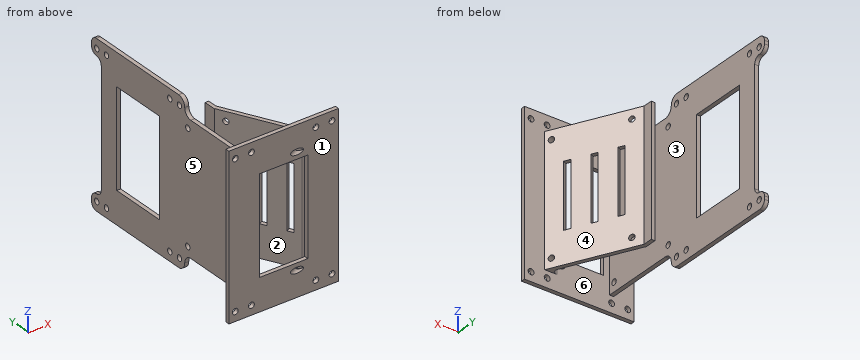
```python
from build123d import *

# Parameters (mm, degrees)
SKETCH_1_W           = 68
SKETCH_1_H           = 100
SKETCH_1_R           = 1.8
EXTRUDE_1_DEPTH      = 2.5
SKETCH_3_W           = 2.5
SKETCH_3_H           = 80
EXTRUDE_2_DEPTH      = 55
SKETCH_4_W           = 30
SKETCH_4_H           = 60
CUT_EXTRUDE_1_DEPTH  = 55
EXTRUDE_3_DEPTH      = 40
EXTRUDE_3_DEPTH_BACK = 40
SKETCH_5_W           = 80
SKETCH_5_H           = 55
EXTRUDE_5_DEPTH      = 2.5
SKETCH_6_R           = 1.8
CUT_EXTRUDE_2_DEPTH  = 2.5
SKETCH_7_R           = 1.8
CUT_EXTRUDE_3_DEPTH  = 2.5
EXTRUDE_START        = 55
SKETCH_8_W           = 2.236067978
SKETCH_8_H           = 80
EXTRUDE_6_DEPTH      = 7.5
SKETCH_10_R          = 1.8
SKETCH_10_W          = 80
SKETCH_10_H          = 3
SKETCH_10_W_2        = 10
SKETCH_10_H_2        = 1.3
SKETCH_10_W_3        = 100
EXTRUDE_7_DEPTH      = 2.5
FILLET_1_R           = 5
FILLET_4_R           = 3
SKETCH_11_R          = 1.8
CUT_EXTRUDE_4_DEPTH  = 30
SKETCH_13_W          = 40
SKETCH_13_H          = 4
CUT_EXTRUDE_5_DEPTH  = 2.5
SKETCH_14_R          = 1.8
CUT_EXTRUDE_6_DEPTH  = 2.5
SKETCH_15_R          = 1.8
EXTRUDE_10_DEPTH     = 2.5
FILLET_6_R           = 4
SKETCH_16_W          = 60
SKETCH_16_H          = 35.254237288
CUT_EXTRUDE_8_DEPTH  = 10


# Some blends are built 0.0001 mm under size
with BuildPart() as part:
    # 草图1 → 凸台-拉伸1 (new body)
    with BuildSketch(Plane(origin=(0, 0, 0), x_dir=(1, 0, 0), z_dir=(0, 1, 0))):
        Rectangle(SKETCH_1_W, SKETCH_1_H)
        with Locations(Location((-30, 44.25, 0), (0, 0, 270))):
            Circle(SKETCH_1_R, mode=Mode.SUBTRACT)
        with Locations(Location((30, 44.25, 0), (0, 0, 270))):
            Circle(SKETCH_1_R, mode=Mode.SUBTRACT)
        with Locations(Location((30, -44.25, 0), (0, 0, 270))):
            Circle(SKETCH_1_R, mode=Mode.SUBTRACT)
        with Locations(Location((-30, -44.25, 0), (0, 0, 270))):
            Circle(SKETCH_1_R, mode=Mode.SUBTRACT)
        with Locations(Location((20, -44.25, 0), (0, 0, 270))):
            Circle(SKETCH_1_R, mode=Mode.SUBTRACT)
        with Locations(Location((20, 44.25, 0), (0, 0, 270))):
            Circle(SKETCH_1_R, mode=Mode.SUBTRACT)
        with Locations(Location((-20, -44.25, 0), (0, 0, 270))):
            Circle(SKETCH_1_R, mode=Mode.SUBTRACT)
        with Locations(Location((-20, 44.25, 0), (0, 0, 270))):
            Circle(SKETCH_1_R, mode=Mode.SUBTRACT)
    extrude(amount=EXTRUDE_1_DEPTH)

    # 草图3 → 凸台-拉伸2 (add)
    with BuildSketch(Plane(origin=(0, 2.5, 0), x_dir=(1, 0, 0), z_dir=(0, 1, 0))):
        with Locations((-20, 0)):
            Rectangle(SKETCH_3_W, SKETCH_3_H)
    extrude(amount=EXTRUDE_2_DEPTH)

    # 草图4 → 切除-拉伸1 (cut)
    with BuildSketch(Plane(origin=(0, 2.5, 0), x_dir=(1, 0, 0), z_dir=(0, 1, 0))):
        Rectangle(SKETCH_4_W, SKETCH_4_H)
    extrude(amount=-CUT_EXTRUDE_1_DEPTH, mode=Mode.SUBTRACT)

    # 草图2 → 凸台-拉伸3 (add, two sides: drawn at the far end of the back side and taken through both)
    with BuildSketch(Plane.XY.offset(-EXTRUDE_3_DEPTH_BACK)):
        Polygon((20, 2.5), (21.5, 2.5), (20, 5.5), align=None)
    extrude(amount=EXTRUDE_3_DEPTH + EXTRUDE_3_DEPTH_BACK)

    # 草图5 → 凸台-拉伸5 (add)
    with BuildSketch(Plane(origin=(18.2, 9.1, 0), x_dir=(0, 0, -1), z_dir=(0.8944271909999156, 0.44721359549995837, 0))):
        with Locations((0, 20.120975674)):
            Rectangle(SKETCH_5_W, SKETCH_5_H)
    extrude(amount=-EXTRUDE_5_DEPTH)

    # 草图6 → 切除-拉伸2 (cut)
    with BuildSketch(Plane.ZY.offset(21.25)):
        with Locations((34.25, 50.7)):
            Circle(SKETCH_6_R)
        with Locations((34.25, 6.2)):
            Circle(SKETCH_6_R)
        with Locations((-34.25, 50.7)):
            Circle(SKETCH_6_R)
        with Locations((-34.25, 6.2)):
            Circle(SKETCH_6_R)
    extrude(amount=-CUT_EXTRUDE_2_DEPTH, mode=Mode.SUBTRACT)

    # 草图7 → 切除-拉伸3 (cut)
    with BuildSketch(Plane(origin=(18.2, 9.1, 0), x_dir=(0, 0, -1), z_dir=(0.8944271909999156, 0.44721359549995837, 0))):
        with Locations(Location((34.25, 40.820975674, 0), (0, 0, 90))):
            Circle(SKETCH_7_R)
        with Locations(Location((-34.25, 40.820975674, 0), (0, 0, 90))):
            Circle(SKETCH_7_R)
        with Locations(Location((-34.25, -3.679024326, 0), (0, 0, 90))):
            Circle(SKETCH_7_R)
        with Locations(Location((34.25, -3.679024326, 0), (0, 0, 90))):
            Circle(SKETCH_7_R)
    extrude(amount=-CUT_EXTRUDE_3_DEPTH, mode=Mode.SUBTRACT)

    # 草图8 → 凸台-拉伸6 (add)
    with BuildSketch(Plane(origin=(0, 2.5, 0), x_dir=(1, 0, 0), z_dir=(0, 1, 0)).offset(EXTRUDE_START)):
        with Locations((-4.214781741, 0)):
            Rectangle(SKETCH_8_W, SKETCH_8_H)
    extrude(amount=-EXTRUDE_6_DEPTH)

    # 草图10 → 凸台-拉伸7 (add)
    # profile 1 of 5: a face of its own
    with BuildSketch(Plane.ZY.offset(21.25)):
        Polygon((50, 120.5), (-50, 120.5), (-50, 54.5), (-40, 54.5), (-40, 57.5), (40, 57.5), (40, 54.5), (50, 54.5), align=None)
        with Locations((-44.25, 57.5)):
            Circle(SKETCH_10_R, mode=Mode.SUBTRACT)
        with Locations((44.25, 57.5)):
            Circle(SKETCH_10_R, mode=Mode.SUBTRACT)
        with Locations((-44.25, 117.5)):
            Circle(SKETCH_10_R, mode=Mode.SUBTRACT)
        with Locations((44.25, 117.5)):
            Circle(SKETCH_10_R, mode=Mode.SUBTRACT)
    # profile 2 of 5: a face of its own
    with BuildSketch(Plane.ZY.offset(21.25)):
        with Locations((0, 56)):
            Rectangle(SKETCH_10_W, SKETCH_10_H)
    # profile 3 of 5: a face of its own
    with BuildSketch(Plane.ZY.offset(21.25)):
        with Locations((-45, 53.85)):
            Rectangle(SKETCH_10_W_2, SKETCH_10_H_2)
    # profile 4 of 5: a face of its own
    with BuildSketch(Plane.ZY.offset(21.25)):
        with Locations((45, 53.85)):
            Rectangle(SKETCH_10_W_2, SKETCH_10_H_2)
    # profile 5 of 5: a face of its own
    with BuildSketch(Plane.ZY.offset(21.25)):
        with Locations((0, 121.15)):
            Rectangle(SKETCH_10_W_3, SKETCH_10_H_2)
    extrude(amount=-EXTRUDE_7_DEPTH)

    # 圆角1
    fillet_1_edges = [part.edges().sort_by_distance(p)[0] for p in [
        (-20, 121.8, -50),
        (-20, 121.8, 50),
        (-20, 53.2, 50),
        (-20, 53.2, -50),
        (-20, 53.2, -40),
        (-20, 53.2, 40),
    ]]
    fillet(fillet_1_edges, radius=FILLET_1_R - 0.0001)  # a hair under: the kernel refuses the full size

    # 圆角4
    # the kernel refuses this fillet: 3 mm, written as the material it adds along each edge
    with BuildSketch(Plane(origin=(18.704915028, 2.5, 40), x_dir=(-1, 0, 0), z_dir=(0, 0, -1))) as fillet_4_piece_1_section:
        with BuildLine():
            CenterArc((FILLET_4_R * 1.61803398875, FILLET_4_R), FILLET_4_R, 153.434948823, 116.565051177)
            Line((FILLET_4_R * 0.72360679775, FILLET_4_R * 1.4472135955), (0, 0))
            Line((0, 0), (FILLET_4_R * 1.61803398875, 0))
        make_face()
    fillet_4_piece_1 = extrude(amount=92.135254916, mode=Mode.PRIVATE)
    fillet_4_piece_1 = split(fillet_4_piece_1, bisect_by=Plane(origin=(14.716283271, 2.568197863, 30), z_dir=(0, 0, 1)), keep=Keep.TOP, mode=Mode.PRIVATE)
    fillet_4_piece_1 = fillet_4_piece_1 - Plane(origin=(14.445615458, 3.109533488, 34.25), x_dir=(-0.44721359549995837, 0.8944271909999156, 0), z_dir=(0.8944271909999156, 0.44721359549995837, 0)) * Cylinder(1.8, 204, mode=Mode.PRIVATE)
    add(fillet_4_piece_1)
    with BuildSketch(Plane(origin=(18.704915028, 2.5, 52.135254916), x_dir=(-1, 0, 0), z_dir=(0, 0, -1))) as fillet_4_piece_2_section:
        with BuildLine():
            CenterArc((FILLET_4_R * 1.61803398875, FILLET_4_R), FILLET_4_R, 153.434948823, 116.565051177)
            Line((FILLET_4_R * 0.72360679775, FILLET_4_R * 1.4472135955), (0, 0))
            Line((0, 0), (FILLET_4_R * 1.61803398875, 0))
        make_face()
    fillet_4_piece_2 = extrude(amount=92.135254916, mode=Mode.PRIVATE)
    fillet_4_piece_2 = split(fillet_4_piece_2, bisect_by=Plane(origin=(17.041037704, 3.56720979, 30), z_dir=(0, 0, -1)), keep=Keep.TOP, mode=Mode.PRIVATE)
    fillet_4_piece_2 = split(fillet_4_piece_2, bisect_by=Plane(origin=(15, 3.56720979, 0), z_dir=(1, 0, 0)), keep=Keep.TOP, mode=Mode.PRIVATE)
    fillet_4_piece_2 = fillet_4_piece_2 - Plane(origin=(16.705023776, 4.239237646, -34.25), x_dir=(-0.44721359549995837, 0.8944271909999156, 0), z_dir=(0.8944271909999156, 0.44721359549995837, 0)) * Cylinder(1.8, 204, mode=Mode.PRIVATE)
    add(fillet_4_piece_2)
    with BuildSketch(Plane(origin=(18.704915028, 2.5, 52.135254916), x_dir=(-1, 0, 0), z_dir=(0, 0, -1))) as fillet_4_piece_3_section:
        with BuildLine():
            CenterArc((FILLET_4_R * 1.61803398875, FILLET_4_R), FILLET_4_R, 153.434948823, 116.565051177)
            Line((FILLET_4_R * 0.72360679775, FILLET_4_R * 1.4472135955), (0, 0))
            Line((0, 0), (FILLET_4_R * 1.61803398875, 0))
        make_face()
    fillet_4_piece_3 = extrude(amount=92.135254916, mode=Mode.PRIVATE)
    fillet_4_piece_3 = split(fillet_4_piece_3, bisect_by=Plane(origin=(14.716283305, 2.568197867, -30), z_dir=(0, 0, -1)), keep=Keep.TOP, mode=Mode.PRIVATE)
    fillet_4_piece_3 = fillet_4_piece_3 - Plane(origin=(14.445615487, 3.109533502, -34.25), x_dir=(-0.44721359549995837, 0.8944271909999156, 0), z_dir=(0.8944271909999156, 0.44721359549995837, 0)) * Cylinder(1.8, 204, mode=Mode.PRIVATE)
    add(fillet_4_piece_3)

    # 草图11 → 切除-拉伸4 (cut)
    with BuildSketch(Plane(origin=(18.2, 9.1, 0), x_dir=(0, 0, -1), z_dir=(0.8944271909999156, 0.44721359549995837, 0))):
        with Locations(Location((-34.25, -3.679024326, 0), (0, 0, 90))):
            Circle(SKETCH_11_R)
        with Locations(Location((34.25, -3.679024326, 0), (0, 0, 90))):
            Circle(SKETCH_11_R)
    extrude(amount=-CUT_EXTRUDE_4_DEPTH, mode=Mode.SUBTRACT)

    # 草图13 → 切除-拉伸5 (cut)
    with BuildSketch(Plane(origin=(18.2, 9.1, 0), x_dir=(0, 0, -1), z_dir=(0.8944271909999156, 0.44721359549995837, 0))):
        with Locations((0, 20.120975674)):
            Rectangle(SKETCH_13_W, SKETCH_13_H)
        with Locations((0, 35.120975674)):
            Rectangle(SKETCH_13_W, SKETCH_13_H)
        with Locations((0, 5.120975674)):
            Rectangle(SKETCH_13_W, SKETCH_13_H)
    extrude(amount=-CUT_EXTRUDE_5_DEPTH, mode=Mode.SUBTRACT)

    # 草图14 → 切除-拉伸6 (cut)
    with BuildSketch(Plane.ZY.offset(21.25)):
        with Locations((-44.25, 65.5)):
            Circle(SKETCH_14_R)
        with Locations((44.25, 65.5)):
            Circle(SKETCH_14_R)
    extrude(amount=-CUT_EXTRUDE_6_DEPTH, mode=Mode.SUBTRACT)

    # 草图15 → 凸台-拉伸10 (add)
    # profile 1 of 4: a face of its own
    with BuildSketch(Plane.ZY.offset(21.25)):
        Polygon((-42.960162103, 121.8), (-40, 121.8), (-40, 129.8), (-50, 129.8), (-50, 121.8), (-45, 121.8), align=None)
        with Locations((-44.25, 125.5)):
            Circle(SKETCH_15_R, mode=Mode.SUBTRACT)
    # profile 2 of 4: a face of its own
    with BuildSketch(Plane.ZY.offset(21.25)):
        Polygon((40, 129.8), (40, 121.8), (44.25, 121.8), (45, 121.8), (50, 121.8), (50, 129.8), align=None)
        with Locations((44.25, 125.5)):
            Circle(SKETCH_15_R, mode=Mode.SUBTRACT)
    # profile 3 of 4: a face of its own
    with BuildSketch(Plane.ZY.offset(21.25)):
        Polygon((-50, 114.760162103), (-42.960162103, 121.8), (-45, 121.8), (-50, 121.8), align=None)
    # profile 4 of 4: a face of its own
    with BuildSketch(Plane.ZY.offset(21.25)):
        Polygon((45, 121.8), (44.25, 121.8), (50, 115.456159587), (50, 121.8), align=None)
    extrude(amount=-EXTRUDE_10_DEPTH)

    # 圆角6
    fillet_6_edges = [part.edges().sort_by_distance(p)[0] for p in [
        (-20, 121.8, 40),
        (-20, 129.8, 40),
        (-20, 129.8, 50),
        (-20, 129.8, -50),
        (-20, 129.8, -40),
        (-20, 121.8, -40),
    ]]
    fillet(fillet_6_edges, radius=FILLET_6_R - 0.0001)  # a hair under: the kernel refuses the full size

    # 草图16 → 切除-拉伸8 (cut)
    with BuildSketch(Plane.ZY.offset(21.25)):
        with Locations((0, 91.5)):
            Rectangle(SKETCH_16_W, SKETCH_16_H)
    extrude(amount=-CUT_EXTRUDE_8_DEPTH, mode=Mode.SUBTRACT)


solid = part.part
```
Here's how the part is built. I have some questions about the finished solid (model axes, mm). Face numbers are marked on the shaded views. A direction names the side the tool comes from. Give positions to 0.01 mm unless a question says otherwise; leave off trailing zeros. Order: outer loops, then holes, each group sorted by start corner. A loop starts at its lowest first (then second) coordinate and runs counter-clockwise, first axis right, second up. Notation, with made-up numbers: (-38, 42.5) -> (-32, 42.5) arc R27 cw to (-32, 67.5) -> close; hole circle Ø8 at (-10.5, -29.75). An arc over 180 degrees is marked (long way). Use CSV: the item, a comma, the result in double quotes. Start each with the question number.
Item 1: Thinking about a two-plate mould opening in X: for the marked faces 4, 5 and 6, which applies, pulls with the +X half, pulls with the -X half, needs draft (parallel to the pull), parting line crosses it, or undercut?
Item 2: Suppose I cut it at B-B (y = 84.5). List the corners of the cut face in (x, z) for me.
Item 3: Suppose I cut it at D-D (y = 65.5). List the corners of the cut face in (x, z) for me, and give its area (3 significant figures).
Item 4: I'm going to push flat-ended pins straight in: P1, Ø2, axis at y = 112, z = -25, coming from the -X side; P2, Ø2.5, axis at x = -3.5, z = 7.5, coming from the +Y side; P3, Ø4.5, axis at x = 14, y = 12, coming from the +Z side. Where does each tip first touch, or does it pass through?
Item 5: If I drill on probe 1 along X at (y, z) = (1.1, -44.25); probe 2 along Y at (x, z) = (-19.55, -34.25); probe 3 along Z at (x, y) = (-20.6, 117.5), over which ranges is the centre line in solid material (lowest first)? Write a range as [from, to].
Item 6: Suppose I cut it at A-A (x = -11). List the corners of the cut face in (y, z) for me.
Item 7: On a 3-axis mill with a long thin cutter (end or side, diameter ignored), from which of +Z, -Z, +X, -X, +Y, -Y can I reach the whole of each face in a straight line? I mean the marked faces 1, 2 and 3. Say none if no direction works.
Item 8: Suppose I cut it at C-C (x = 30). List the corners of the cut face in (y, z) for me.
Answer block:
1,face 4,"pulls with the +X half"
1,face 5,"pulls with the -X half"
1,face 6,"undercut"
2,outline,"(-21.25, -50) -> (-18.75, -50) -> (-18.75, -30) -> (-21.25, -30) -> close; (-21.25, 30) -> (-18.75, 30) -> (-18.75, 50) -> (-21.25, 50) -> close"
3,outline,"(-21.25, -50) -> (-18.75, -50) -> (-18.75, -46.05) -> (-21.25, -46.05) -> close; (-21.25, -42.45) -> (-18.75, -42.45) -> (-18.75, 42.45) -> (-21.25, 42.45) -> close; (-21.25, 46.05) -> (-18.75, 46.05) -> (-18.75, 50) -> (-21.25, 50) -> close"
3,area,"232 mm^2"
4,P1,"stops at x = -21.25"
4,P2,"stops at y = 57.5"
4,P3,"stops at z = 40"
5,probe 1,"x = [-34, -31.8], [-28.2, -21.8], [-18.2, 18.2], [21.8, 28.2], [31.8, 34]"
5,probe 2,"y = [0, 4.4], [8, 48.9], [52.5, 121.8]"
5,probe 3,"z = [-50, -46.05], [-42.45, 42.45], [46.05, 50]"
6,outline,"(0, -50) -> (2.5, -50) -> (2.5, -30) -> (0, -30) -> close; (0, 30) -> (2.5, 30) -> (2.5, 50) -> (0, 50) -> close"
7,face 1,"+Z, -Z, +X, -X, -Y"
7,face 2,"+Z, -Z"
7,face 3,"+Z, -Z, +Y"
8,outline,"(0, -50) -> (2.5, -50) -> (2.5, -46.05) -> (0, -46.05) -> close; (0, -42.45) -> (2.5, -42.45) -> (2.5, 42.45) -> (0, 42.45) -> close; (0, 46.05) -> (2.5, 46.05) -> (2.5, 50) -> (0, 50) -> close"
